```python
from build123d import *

# Parameters (mm, degrees)
BASPROSKE_W         = 10
BASPROSKE_H         = 10.625
TOOTHCUT_DEPTH      = 19.049411348
TEETHCUTS_COUNT     = 15
TEETHCUTS_ANGLE     = 336
BORSKE_R            = 2
BORE_DEPTH          = 50.0000508
SKETCH1_R           = 2.2
CUT_EXTRUDE2_DEPTH  = 10
BOSS_EXTRUDE1_DEPTH = 10


with BuildPart() as part:
    # BasProSke → Base-Revolve (revolve)
    with BuildSketch(Plane(origin=(0, 0, 0), x_dir=(1, 0, 0), z_dir=(0, 1, 0)), mode=Mode.PRIVATE) as base_revolve_sk:
        with Locations((5, 5.3125)):
            Rectangle(BASPROSKE_W, BASPROSKE_H)
    revolve(base_revolve_sk.sketch.rotate(Axis((-10, 0, 0), (1, 0, 0)), 180), axis=Axis((-10, 0, 0), (1, 0, 0)))

    # TooCutSke → ToothCut (cut, through all)
    with BuildSketch(Plane(origin=(0, 0, 0), x_dir=(0, 0, -1), z_dir=(1, 0, 0))):
        with BuildLine():
            ThreePointArc((0.660831632, 7.78349753), (0, 7.8115), (-0.660831632, 7.78349753))
            ThreePointArc((-0.660831632, 7.78349753), (-1.031814994, 9.260718016), (-1.959681305, 10.46855622))
            ThreePointArc((-1.959681305, 10.46855622), (0, 10.6504), (1.959681305, 10.46855622))
            ThreePointArc((1.959681305, 10.46855622), (1.031814994, 9.260718016), (0.660831632, 7.78349753))
        make_face()
    toothcut = extrude(amount=TOOTHCUT_DEPTH, mode=Mode.SUBTRACT)

    # TeethCuts: ToothCut ×15 about axis
    teethcuts_axis = Axis((-10, 0, 0), (1, 0, 0))
    for i in range(1, TEETHCUTS_COUNT):
        add(toothcut.rotate(teethcuts_axis, i * TEETHCUTS_ANGLE / (TEETHCUTS_COUNT - 1)), mode=Mode.SUBTRACT)

    # BorSke → Bore (cut, symmetric)
    with BuildSketch(Plane(origin=(0, 0, 0), x_dir=(0, 0, -1), z_dir=(1, 0, 0))):
        with Locations(Location((0, 0, 0), (0, 0, 180))):
            Circle(BORSKE_R)
    extrude(amount=BORE_DEPTH, both=True, mode=Mode.SUBTRACT)

    # Sketch1 → Cut-Extrude2 (cut)
    with BuildSketch(Plane(origin=(10, 0, 0), x_dir=(0, 0, -1), z_dir=(1, 0, 0))):
        Circle(SKETCH1_R)
    extrude(amount=-CUT_EXTRUDE2_DEPTH, mode=Mode.SUBTRACT)

    # Sketch4 → Boss-Extrude1 (add)
    with BuildSketch(Plane(origin=(10, 0, 0), x_dir=(0, 0, -1), z_dir=(1, 0, 0))):
        with BuildLine():
            ThreePointArc((1.609347694, 1.5), (0, 2.2), (-1.609347694, 1.5))
            Line((-1.609347694, 1.5), (1.609347694, 1.5))
        make_face()
    extrude(amount=-BOSS_EXTRUDE1_DEPTH)


solid = part.part
```
Source: CAD feature listing. Evaluate the final solid. Frame: model axes, mm. A direction names the side the tool comes from. Give positions to 0.01 mm unless a question says otherwise; leave off trailing zeros. Order: outer loops, then holes, each group sorted by start corner. A loop starts at its lowest first (then second) coordinate and runs counter-clockwise, first axis right, second up.
(1) Section query B-B (y = -1.75). Return the cut outline in (x, z), plus the area to 3 significant figures.
(2) Section query C-C (y = -8.25). Return the cut outline in (x, z), plus the area to 3 significant figures.
(3) Material intervals for line 1 along Y through (x, z) = (7.25, 1.5); line 2 along Y through (x, z) = (6.25, 0) (1 decimal); line 3 along Y through (x, z) = (9.5, -9.25), sorted ascending.
(4) Access query for faces 1 (the face through (4.93, -6.87, -6.25)), 2 (the face through (4.93, 6.929, -6.177)), 3 (the face through (5, 1.5, 0)), 4 (the face through (4.93, 3.847, 8.492)). Directions: +Z, -Z, +X, -X, +Y, -Y. A direction counts if a zero-diameter tool reaches every point of the face in a straight line with its end or side. Return the directions, or none.
(5) Section query D-D (y = -4.75). Return the cut outline in (x, z).
(6) Section query A-A (z = 0). Return the cut outline in (x, y) (1 decimal), plus the area to 3 significant figures.
(7) Contact query for flat-ended pins moving along their axis: P1, Ø2, axis at x = 9, z = -6.5, coming from the +Y side; P2, Ø3, axis at x = 4, z = 4.5, coming from the -Y side; P3, Ø1, axis at x = 8, y = -7, coming from the +Z side. Output: stop coordinate, or through.
Outcome:
1. outline: (0, -8.64) - (10, -8.64) - (10, -1.33) - (0, -1.33) - close; (0, 1.33) - (10, 1.33) - (10, 8.64) - (0, 8.64) - close
1. area: 146 mm2
2. outline: (0, -4.63) - (10, -4.63) - (10, -2.56) - (0, -2.56) - close; (0, -1.02) - (10, -1.02) - (10, 1.02) - (0, 1.02) - close; (0, 2.56) - (10, 2.56) - (10, 4.63) - (0, 4.63) - close
2. area: 62.0 mm2
3. line 1: y = -7.67 to -1.61, 1.5 to 10
3. line 2: y = -10.6 to -2.2, 1.5 to 7.8
3. line 3: y = -3.72 to -2.09, 0.03 to 1.86, 4.88 to 5.23
4. face 1: +X, -X, -Y
4. face 2: -Z, +X, -X
4. face 3: +X, -X
4. face 4: +Z, +X, -X
5. outline: (0, -6.8) - (10, -6.8) - (10, 6.8) - (0, 6.8) - close
6. outline: (0, -10.6) - (10, -10.6) - (10, -2.2) - (0, -2.2) - close; (0, 1.5) - (10, 1.5) - (10, 7.8) - (0, 7.8) - close
6. area: 147 mm2
7. P1: stops at y = 8.76
7. P2: stops at y = -9.82
7. P3: stops at z = 8.08
